The listing builds one solid part. Answer for the finished solid, in the listing's coordinates (mm). A direction names the side the tool comes from. Round coordinates to 2 decimals unless told otherwise and drop trailing zeros. Write each loop counter-clockwise with the first axis right and the second up, starting at its lowest first coordinate (ties: lowest second). Pieces come first, ordered by that corner, then holes.
Item 1: Find section B-B on y = 5.5. Give the number of separate pieces and of enclosed holes in the cut face, then the cut area to 3 significant figures.
Item 2: For a pull along Z with two mould halves and no side action, classify faces 6 (the face through (-10.5, 5.6, 19.9)), 7 (the face through (6.7, 12.1, 0.4)), 8 (the face through (-0.1, 12, -29.3)), 9 (the face through (-5.5, 4, -4)) as +Z half, -Z half, draft (parallel to the pull), parting line (faces both ways), or undercut.
Item 3: A tool of negligible diameter and unlimited length cuts with its end or side. For faces 1 (the face through (2, 11, -7)), 2 (the face through (6, 4, 13.8)), 3 (the face through (-2.689, 11.222, 22.575)), 4 (the face through (-6.8, 12, 0.2)), 5 (the face through (-10.5, 5.6, -19.9)), from which of +Z, -Z, +X, -X, +Y, -Y can it reach the whole face along a straight path? Write none if from no direction.
Item 4: Find section C-C on z = -7.25. Give the vertices of the cut face in (x, y), then the cut area to 3 significant figures.
Item 5: Each of these flat-tipped pins is pushed along its axis until it touches: pin 1 (2.5 mm diameter, centred on x = -4, z = 20.5, fed in from +Y); pin 2 (1.6 mm diameter, centred on y = 6.5, z = -28, fed in from -X); pin 3 (1.5 mm diameter, centred on x = -7.5, y = 2.5, fed in from -Z). Where does it stop, or does it pass through?
Item 6: Find section A-A on z = -20. Give the vertices of the cut face in (x, y), then the cut area to 3 significant figures.
Item 7: Find the intervals of material crossed by probe 1 along Z at (x, y) = (-3.5, 4.25); probe 2 along X at (y, z) = (9.6, -7.25); probe 3 along Z at (x, y) = (-3.25, 8.25), in increasing order.
Item 8: Find section D-D on z = 20. Give the vertices of the cut face in (x, y).
```python
from build123d import *

# Parameters (mm, degrees)
SKETCH1_W               = 15
SKETCH1_H               = 60
SKETCH1_R               = 1.65
BOSS_EXTRUDE1_DEPTH     = 12.8
CUT_EXTRUDE3_DEPTH      = 34.467745667
CUT_EXTRUDE3_DEPTH_BACK = 8
SKETCH5_W               = 13
SKETCH5_H               = 13
SKETCH6_R               = 1.45
CUT_EXTRUDE4_DEPTH      = 3
SKETCH8_R               = 2.7
CUT_EXTRUDE6_DEPTH      = 3.2
SKETCH9_W               = 4
SKETCH9_H               = 19.5
CUT_EXTRUDE7_DEPTH      = 2
SKETCH10_W              = 12.4
SKETCH10_H              = 8.4
CUT_EXTRUDE8_DEPTH      = 3
CUT_EXTRUDE9_DEPTH      = 0.6
FILLET1_SIZE            = 0.5
BOSS_EXTRUDE2_DEPTH     = 12.8
CHAMFER2_SIZE           = 1.5
FILLET3_SIZE            = 1
CHAMFER3_SIZE           = 0.6


with BuildPart() as part:
    # Sketch1 → Boss-Extrude1 (new body)
    with BuildSketch(Plane(origin=(0, 0, 0), x_dir=(1, 0, 0), z_dir=(0, 1, 0))):
        Rectangle(SKETCH1_W, SKETCH1_H)
        with Locations(Location((-3.5, 20, 0), (0, 0, 270))):
            Circle(SKETCH1_R, mode=Mode.SUBTRACT)
        with Locations(Location((-3.5, -20, 0), (0, 0, 270))):
            Circle(SKETCH1_R, mode=Mode.SUBTRACT)
    extrude(amount=BOSS_EXTRUDE1_DEPTH)

    # Sketch5 → Cut-Extrude3 (cut, two sides: drawn at the far end of the back side and taken through both)
    with BuildSketch(Plane.XZ.offset(-CUT_EXTRUDE3_DEPTH_BACK)):
        with Locations((1, -4)):
            Rectangle(SKETCH5_W, SKETCH5_H)
    extrude(amount=CUT_EXTRUDE3_DEPTH + CUT_EXTRUDE3_DEPTH_BACK, mode=Mode.SUBTRACT)

    # Sketch6 → Cut-Extrude4 (cut)
    with BuildSketch(Plane.XZ.offset(-8)):
        with Locations(Location((2.5, -0.75, 0), (0, 0, 270))):
            Circle(SKETCH6_R)
        with Locations(Location((2.5, -7.25, 0), (0, 0, 90))):
            Circle(SKETCH6_R)
    extrude(amount=-CUT_EXTRUDE4_DEPTH, mode=Mode.SUBTRACT)

    # Sketch8 → Cut-Extrude6 (cut)
    with BuildSketch(Plane(origin=(0, 12.8, 0), x_dir=(1, 0, 0), z_dir=(0, 1, 0))):
        with Locations(Location((-3.5, 20, 0), (0, 0, 270))):
            Circle(SKETCH8_R)
        with Locations(Location((-3.5, -20, 0), (0, 0, 270))):
            Circle(SKETCH8_R)
    extrude(amount=-CUT_EXTRUDE6_DEPTH, mode=Mode.SUBTRACT)

    # Sketch9 → Cut-Extrude7 (cut)
    with BuildSketch(Plane.XZ):
        with Locations((0.5, -20.25)):
            Rectangle(SKETCH9_W, SKETCH9_H)
    extrude(amount=-CUT_EXTRUDE7_DEPTH, mode=Mode.SUBTRACT)

    # Sketch10 → Cut-Extrude8 (cut)
    with BuildSketch(Plane(origin=(7.5, 0, 0), x_dir=(0, 0, -1), z_dir=(1, 0, 0))):
        with Locations((-20, 4.2)):
            Rectangle(SKETCH10_W, SKETCH10_H)
        with Locations((20, 4.2)):
            Rectangle(SKETCH10_W, SKETCH10_H)
    extrude(amount=-CUT_EXTRUDE8_DEPTH, mode=Mode.SUBTRACT)

    # Sketch11 → Cut-Extrude9 (cut)
    with BuildSketch(Plane(origin=(0, 12.8, 0), x_dir=(1, 0, 0), z_dir=(0, 1, 0))):
        Polygon((-3.050724638, -5), (-3.050724638, 5), (-1.166666667, 5), (-1.166666667, -3.405797101), (3.036231884, -3.405797101), (3.036231884, -5), align=None)
    extrude(amount=-CUT_EXTRUDE9_DEPTH, mode=Mode.SUBTRACT)

    # Fillet1
    # a fillet whose section is not a circle: 0.5 mm, written as the material it adds along each edge
    with BuildSketch(Plane(origin=(7.5, 8.4, 26.2), x_dir=(0, 0, -1), z_dir=(-1, 0, 0)), Plane(origin=(7.5, 8.4, 13.8), x_dir=(0, -1, 0), z_dir=(-1, 0, 0)), Plane(origin=(7.5, 8.4, -13.8), x_dir=(0, 0, -1), z_dir=(-1, 0, 0)), Plane(origin=(7.5, 8.4, -26.2), x_dir=(0, -1, 0), z_dir=(-1, 0, 0))) as fillet1_piece_1:
        with BuildLine():
            Bezier((FILLET1_SIZE, 0), (0, 0), (0, FILLET1_SIZE), weights=[1, 1, 1])
            Line((0, FILLET1_SIZE), (0, 0))
            Line((0, 0), (FILLET1_SIZE, 0))
        make_face()
    extrude(amount=4.25)

    # Sketch12 → Boss-Extrude2 (add)
    with BuildSketch(Plane(origin=(0, 0, 0), x_dir=(1, 0, 0), z_dir=(0, 1, 0))):
        with BuildLine():
            Line((-7.5, 25.744562647), (-7.5, 14.255437353))
            ThreePointArc((-7.5, 14.255437353), (-10.5, 20), (-7.5, 25.744562647))
        make_face()
        with BuildLine():
            Line((-7.5, -25.744562647), (-7.5, -14.255437353))
            ThreePointArc((-7.5, -14.255437353), (-10.5, -20), (-7.5, -25.744562647))
        make_face()
    extrude(amount=BOSS_EXTRUDE2_DEPTH)

    # Chamfer2
    chamfer2_edges = [part.edges().sort_by_distance(p)[0] for p in [
        (7.5, 12.8, 0),
        (-7.5, 12.8, 0),
        (0, 12.8, -30),
        (-7.5, 12.8, 27.872281323),
        (-10.5, 12.8, -20),
        (-10.5, 12.8, 20),
        (-7.5, 12.8, -27.872281323),
        (0, 12.8, 30),
    ]]
    chamfer(chamfer2_edges, length=CHAMFER2_SIZE)

    # Fillet3
    # a fillet whose section is not a circle: 1 mm, written as the material it takes off along each edge
    with BuildSketch(Plane(origin=(-7.5, -2.5, -30), x_dir=(1, 0, 0), z_dir=(0, 1, 0)), Plane(origin=(7.5, -2.5, -30), x_dir=(0, 0, 1), z_dir=(0, 1, 0))) as fillet3_piece_1:
        with BuildLine():
            Bezier((FILLET3_SIZE, 0), (0, 0), (0, -FILLET3_SIZE), weights=[1, 1, 1])
            Line((0, -FILLET3_SIZE), (0, 0))
            Line((0, 0), (FILLET3_SIZE, 0))
        make_face()
    extrude(amount=16.3, mode=Mode.SUBTRACT)
    with BuildSketch(Plane(origin=(7.5, -2.5, 30), x_dir=(0, 0, -1), z_dir=(0, 1, 0)), Plane(origin=(-7.5, -2.5, 30), x_dir=(1, 0, 0), z_dir=(0, 1, 0))) as fillet3_piece_2:
        with BuildLine():
            Bezier((FILLET3_SIZE, 0), (0, 0), (0, FILLET3_SIZE), weights=[1, 1, 1])
            Line((0, FILLET3_SIZE), (0, 0))
            Line((0, 0), (FILLET3_SIZE, 0))
        make_face()
    extrude(amount=16.3, mode=Mode.SUBTRACT)

    # Chamfer3
    chamfer3_edges = [part.edges().sort_by_distance(p)[0] for p in [
        (2.5, 8, 0.7),
        (2.5, 8, -8.7),
    ]]
    chamfer(chamfer3_edges, length=CHAMFER3_SIZE)


solid = part.part
```
Check values:
1. separate pieces: 1
1. enclosed holes: 2
1. area: 687 mm2
2. face 6: undercut
2. face 7: draft
2. face 8: -Z half
2. face 9: undercut
3. face 1: -Y
3. face 2: +X, -Y
3. face 3: +Y
3. face 4: -X, +Y
3. face 5: -X, +Y, -Y
4. outline: (-7.5, 0) - (-5.5, 0) - (-5.5, 8) - (0.45, 8) - (1.05, 8.6) - (1.05, 11) - (3.95, 11) - (3.95, 8.6) - (4.55, 8) - (7.5, 8) - (7.5, 11.3) - (6, 12.8) - (-6, 12.8) - (-7.5, 11.3) - close
4. area: 76.7 mm2
5. pin 1: stops at y = 9.6
5. pin 2: stops at x = -7.5
5. pin 3: stops at z = -29.98
6. outline: (-10.5, 0) - (-5.15, 0) - (-5.15, 9.6) - (-6.2, 9.6) - (-6.2, 12.8) - (-9, 12.8) - (-10.5, 11.3) - close; (-1.85, 0) - (-1.5, 0) - (-1.5, 2) - (2.5, 2) - (2.5, 0) - (4.5, 0) - (4.5, 8.4) - (7.5, 8.4) - (7.5, 11.3) - (6, 12.8) - (-0.8, 12.8) - (-0.8, 9.6) - (-1.85, 9.6) - close
6. area: 146 mm2
7. probe 1: z = -30 to -21.65, -18.35 to -10.5, 2.5 to 18.35, 21.65 to 30
7. probe 2: x = -7.5 to 1.05, 3.95 to 7.5
7. probe 3: z = -30 to -21.63, -18.37 to 18.37, 21.63 to 30
8. outline: (-10.5, 0) - (-5.15, 0) - (-5.15, 9.6) - (-6.2, 9.6) - (-6.2, 12.8) - (-9, 12.8) - (-10.5, 11.3) - close; (-1.85, 0) - (4.5, 0) - (4.5, 8.4) - (7.5, 8.4) - (7.5, 11.3) - (6, 12.8) - (-0.8, 12.8) - (-0.8, 9.6) - (-1.85, 9.6) - close
